Part model, mm, in its own coordinate system. Face numbers are marked on the shaded views. Give positions to 0.01 mm unless a question says otherwise; leave off trailing zeros. Order: outer loops, then holes, each group sorted by start corner. A loop starts at its lowest first (then second) coordinate and runs counter-clockwise, first axis right, second up. Notation, with made-up numbers: (67.5, -16.75) - (74.5, -16.75) arc R29 ccw to (74.5, 5.25) - close; hole circle Ø6 at (31.5, -19.75). An arc over 180 degrees is marked (long way). One line per item, written item: value.
```python
from build123d import *

# Parameters (mm, degrees)
SKETCH1_R           = 2
BOSS_EXTRUDE1_DEPTH = 1
BOSS_EXTRUDE2_DEPTH = 11
SKETCH3_W           = 34.23
SKETCH3_H           = 19.064187878
CUT_EXTRUDE2_DEPTH  = 1


with BuildPart() as part:
    # Sketch1 → Boss-Extrude1 (new body)
    with BuildSketch(Plane(origin=(0, 0, 0), x_dir=(1, 0, 0), z_dir=(0, 1, 0))):
        with BuildLine():
            ThreePointArc((-44.4, -53.4), (-50.763961031, -50.763961031), (-53.4, -44.4))
            Line((-53.4, -44.4), (-53.4, 44.4))
            ThreePointArc((-53.4, 44.4), (-50.763961031, 50.763961031), (-44.4, 53.4))
            Line((-44.4, 53.4), (44.4, 53.4))
            ThreePointArc((44.4, 53.4), (50.763961031, 50.763961031), (53.4, 44.4))
            Line((53.4, 44.4), (53.4, -44.4))
            ThreePointArc((53.4, -44.4), (50.763961031, -50.763961031), (44.4, -53.4))
            Line((44.4, -53.4), (-44.4, -53.4))
        make_face()
        with BuildLine():
            Line((-29, -25), (-29, 25))
            ThreePointArc((-29, 25), (-27.828427125, 27.828427125), (-25, 29))
            Line((-25, 29), (25, 29))
            ThreePointArc((25, 29), (27.828427125, 27.828427125), (29, 25))
            Line((29, 25), (29, -25))
            ThreePointArc((29, -25), (27.828427125, -27.828427125), (25, -29))
            Line((25, -29), (-25, -29))
            ThreePointArc((-25, -29), (-27.828427125, -27.828427125), (-29, -25))
        make_face(mode=Mode.SUBTRACT)
        with BuildLine():
            ThreePointArc((-29, 25), (-27.828427125, 27.828427125), (-25, 29))
            Line((-25, 29), (25, 29))
            ThreePointArc((25, 29), (27.828427125, 27.828427125), (29, 25))
            Line((29, 25), (29, -25))
            ThreePointArc((29, -25), (27.828427125, -27.828427125), (25, -29))
            Line((25, -29), (-25, -29))
            ThreePointArc((-25, -29), (-27.828427125, -27.828427125), (-29, -25))
            Line((-29, -25), (-29, 25))
        make_face()
        with Locations((25, -25)):
            Circle(SKETCH1_R, mode=Mode.SUBTRACT)
        with Locations((25, 25)):
            Circle(SKETCH1_R, mode=Mode.SUBTRACT)
        with Locations((-25, 25)):
            Circle(SKETCH1_R, mode=Mode.SUBTRACT)
        with Locations((-25, -25)):
            Circle(SKETCH1_R, mode=Mode.SUBTRACT)
    extrude(amount=BOSS_EXTRUDE1_DEPTH)

    # Sketch1<5> → Boss-Extrude2 (add)
    with BuildSketch(Plane(origin=(0, 0, 0), x_dir=(1, 0, 0), z_dir=(0, 1, 0))):
        with BuildLine():
            ThreePointArc((-54.4, 44.4), (-51.471067812, 51.471067812), (-44.4, 54.4))
            Line((-44.4, 54.4), (44.4, 54.4))
            ThreePointArc((44.4, 54.4), (51.471067812, 51.471067812), (54.4, 44.4))
            Line((54.4, 44.4), (54.4, -44.4))
            ThreePointArc((54.4, -44.4), (51.471067812, -51.471067812), (44.4, -54.4))
            Line((44.4, -54.4), (-44.4, -54.4))
            ThreePointArc((-44.4, -54.4), (-51.471067812, -51.471067812), (-54.4, -44.4))
            Line((-54.4, -44.4), (-54.4, 44.4))
        make_face()
        with BuildLine():
            Line((-44.4, -53.4), (44.4, -53.4))
            ThreePointArc((44.4, -53.4), (50.763961031, -50.763961031), (53.4, -44.4))
            Line((53.4, -44.4), (53.4, 44.4))
            ThreePointArc((53.4, 44.4), (50.763961031, 50.763961031), (44.4, 53.4))
            Line((44.4, 53.4), (-44.4, 53.4))
            ThreePointArc((-44.4, 53.4), (-50.763961031, 50.763961031), (-53.4, 44.4))
            Line((-53.4, 44.4), (-53.4, -44.4))
            ThreePointArc((-53.4, -44.4), (-50.763961031, -50.763961031), (-44.4, -53.4))
        make_face(mode=Mode.SUBTRACT)
    extrude(amount=BOSS_EXTRUDE2_DEPTH)

    # Sketch3 → Cut-Extrude2 (cut)
    with BuildSketch(Plane(origin=(0, 0, 54.4), x_dir=(-1, 0, 0), z_dir=(0, 0, -1))):
        with Locations((-2.557601794, 10.532093939)):
            Rectangle(SKETCH3_W, SKETCH3_H)
    extrude(amount=CUT_EXTRUDE2_DEPTH, mode=Mode.SUBTRACT)


solid = part.part
```
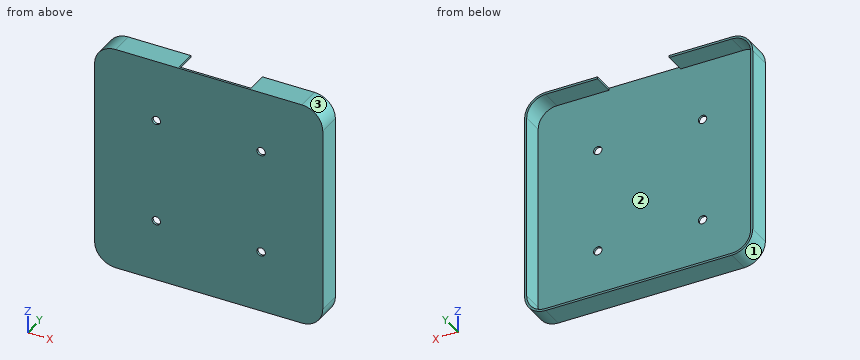
1) Mould opens along Z. For the marked faces 1, 2 and 3 say: released by +Z, released by -Z, zero draft, split by the parting line, or undercut.
Outcome:
face 1: released by -Z
face 2: undercut
face 3: released by +Z
2) Cut at D-D, the plane z = -5. Give the cut face in (x, y).
Outcome:
outline: (-54.4, 0) - (54.4, 0) - (54.4, 11) - (53.4, 11) - (53.4, 1) - (-53.4, 1) - (-53.4, 11) - (-54.4, 11) - close
3) Cut at B-B, the plane z = -25. Give the cut face in (x, y).
Outcome:
outline: (-54.4, 0) - (-27, 0) - (-27, 1) - (-53.4, 1) - (-53.4, 11) - (-54.4, 11) - close; (-23, 0) - (23, 0) - (23, 1) - (-23, 1) - close; (27, 0) - (54.4, 0) - (54.4, 11) - (53.4, 11) - (53.4, 1) - (27, 1) - close
4) Cut at A-A, the plane x = 25. Give the cut face in (y, z), then the cut area to 3 significant figures.
Outcome:
outline: (0, -54.4) - (11, -54.4) - (11, -53.4) - (1, -53.4) - (1, -27) - (0, -27) - close; (0, -23) - (1, -23) - (1, 23) - (0, 23) - close; (0, 27) - (1, 27) - (1, 53.4) - (11, 53.4) - (11, 54.4) - (0, 54.4) - close
area: 121 mm^2
5) Pin check, flat tips, straight feed: pin 1 (1.1 mm diameter, centred on y = 7.5, z = 54, fed in from +X); pin 2 (3 mm diameter, centred on x = -25, z = -25, fed in from +Y); pin 3 (3 mm diameter, centred on x = 42.5, z = -25.5, fed in from +Y). Stop position of each tip, or through.
Outcome:
pin 1: stops at x = 48.65
pin 2: passes through
pin 3: stops at y = 1
6) Drill centre lines: line 1 along X through (y, z) = (0.8, 25); line 2 along X through (y, z) = (8, 19). Where is each one in solid material? Low to high. Write a range as from..to.
Outcome:
line 1: x = -54.4..-27, -23..23, 27..54.4
line 2: x = -54.4..-53.4, 53.4..54.4
7) Cut at C-C, the plane y = 3. Give the cut face in (x, z), then the cut area to 3 significant figures.
Outcome:
outline: (-54.4, -44.4) arc R10 ccw to (-44.4, -54.4) - (44.4, -54.4) arc R10 ccw to (54.4, -44.4) - (54.4, 44.4) arc R10 ccw to (44.4, 54.4) - (19.67, 54.4) - (19.67, 53.4) - (44.4, 53.4) arc R9 cw to (53.4, 44.4) - (53.4, -44.4) arc R9 cw to (44.4, -53.4) - (-44.4, -53.4) arc R9 cw to (-53.4, -44.4) - (-53.4, 44.4) arc R9 cw to (-44.4, 53.4) - (-14.56, 53.4) - (-14.56, 54.4) - (-44.4, 54.4) arc R10 ccw to (-54.4, 44.4) - close
area: 381 mm^2
